For this review, take the finished solid that the model builds, in its own axes (mm). Face numbers are marked on the shaded views. A direction names the side the tool comes from. Give positions to 0.01 mm unless a question says otherwise; leave off trailing zeros. Write each loop counter-clockwise with the first axis right and the second up, starting at its lowest first coordinate (ties: lowest second). Pieces come first, ordered by that corner, then holes. Notation, with made-up numbers: (45, 36) -> (72, 36) arc R15 ccw to (72, 50) -> close; hole circle Ø6 at (-31, -4.75). An arc over 180 degrees is marked (long way). Return JSON: item names as keys, results as strings.
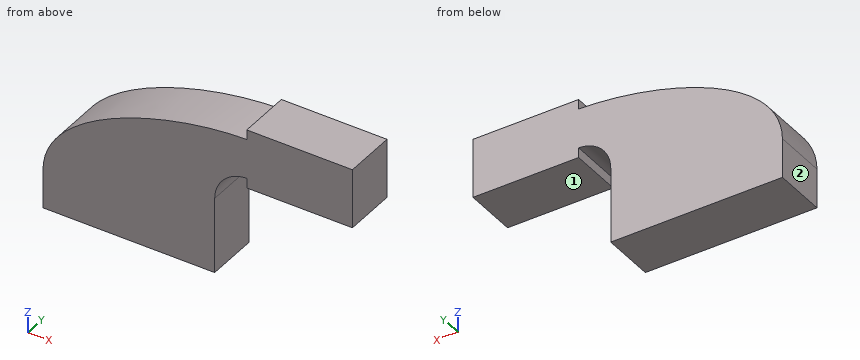
from build123d import *

# Parameters (mm, degrees)
F0_W     = 25.4
F0_H     = 28.575
F1_DEPTH = 25.4


with BuildPart() as f1:
    # F0 (on Front) → F1 (new body)
    with BuildSketch(Plane.XZ):
        Polygon((41.275, -9.525), (41.275, 9.525), (22.225, 9.525), (-41.275, 9.525), (-41.275, -9.525), align=None)
        with BuildLine():
            Line((22.225, 9.525), (41.275, 9.525))
            Line((41.275, 9.525), (41.275, 27.0002))
            ThreePointArc((41.275, 27.0002), (45.7700842218, 38.0687654844), (56.7097265362, 42.869093606))
            Line((56.7097265362, 42.869093606), (56.7097265362, 61.9219276004))
            add(Edge.make_bspline(
                [(56.5976430534, 61.9208318214), (56.6350247317, 61.9212149579), (56.6723859179, 61.921580219), (56.7097265362, 61.9219276004)],
                knots=[110.9664964384, 110.9664964384, 110.9664964384, 110.9664964384, 111.075437095, 111.075437095, 111.075437095, 111.075437095], degree=3))
            ThreePointArc((56.5976430534, 61.9208318214), (32.2597740934, 51.4998383508), (22.225, 27.0002))
            Line((22.225, 27.0002), (22.225, 9.525))
        make_face()
        with BuildLine():
            Line((-41.275, 9.525), (22.225, 9.525))
            Line((22.225, 9.525), (22.225, 27.0002))
            ThreePointArc((22.225, 27.0002), (32.2597740934, 51.4998383508), (56.5976430534, 61.9208318214))
            add(Edge.make_bspline(
                [(-41.275, 9.525), (-40.8172895576, 42.5938186475), (18.5208221845, 61.5305705249), (56.5976430534, 61.9208318214)],
                knots=[0, 0, 0, 0, 110.9664964384, 110.9664964384, 110.9664964384, 110.9664964384], degree=3))
        make_face()
        with BuildLine():
            Line((56.7097265362, 61.9219276004), (56.7097265362, 42.869093606))
            Line((56.7097265362, 42.869093606), (56.7097265362, 38.1))
            Line((56.7097265362, 38.1), (82.1097265362, 38.1))
            Line((82.1097265362, 38.1), (82.1097265362, 66.675))
            Line((82.1097265362, 66.675), (56.7097265362, 66.675))
            Line((56.7097265362, 66.675), (56.7097265362, 61.9224247899))
            ThreePointArc((56.7097265362, 61.9224247899), (56.9298588949, 61.9245061906), (57.15, 61.9252))
            add(Edge.make_bspline(
                [(56.7097265362, 61.9219276004), (56.856805001, 61.9232958778), (57.0035643669, 61.9243867627), (57.15, 61.9252)],
                knots=[111.075437095, 111.075437095, 111.075437095, 111.075437095, 111.5045361635, 111.5045361635, 111.5045361635, 111.5045361635], degree=3))
        make_face()
        with BuildLine():
            ThreePointArc((56.7097265362, 61.9224247899), (56.6536841557, 61.9216732734), (56.5976430534, 61.9208318214))
            add(Edge.make_bspline(
                [(56.5976430534, 61.9208318214), (56.6350247317, 61.9212149579), (56.6723859179, 61.921580219), (56.7097265362, 61.9219276004)],
                knots=[110.9664964384, 110.9664964384, 110.9664964384, 110.9664964384, 111.075437095, 111.075437095, 111.075437095, 111.075437095], degree=3))
            Line((56.7097265362, 61.9219276004), (56.7097265362, 61.9224247899))
        make_face()
        with BuildLine():
            Line((56.7097265362, 61.9224247899), (56.7097265362, 61.9219276004))
            add(Edge.make_bspline(
                [(56.7097265362, 61.9219276004), (56.856805001, 61.9232958778), (57.0035643669, 61.9243867627), (57.15, 61.9252)],
                knots=[111.075437095, 111.075437095, 111.075437095, 111.075437095, 111.5045361635, 111.5045361635, 111.5045361635, 111.5045361635], degree=3))
            ThreePointArc((57.15, 61.9252), (56.9298588949, 61.9245061906), (56.7097265362, 61.9224247899))
        make_face()
        with Locations((94.8097265362, 52.3875)):
            Rectangle(F0_W, F0_H)
    extrude(amount=F1_DEPTH)


solid = f1.part
1. For the marked faces 1 and 2, list the 3-axis set-ups (+Z, -Z, +X, -X, +Y, -Y) from which the entire face can be reached by the end or side of a thin tool; tool diameter is ignored.
Results found:
{"face 1": "-Z, +X, +Y, -Y", "face 2": "+Z, -Z, -X, +Y, -Y"}
2. To check wall thickness, follow probe 1 along Z at (x, y) = (93.5, -16) (3 decimals); probe 2 along X at (y, z) = (-6, 9.5) (3 decimals); probe 3 along X at (y, z) = (-9.5, 39). State the ranges of each line that lie inside material, in increasing order.
Results found:
{"probe 1": "z = 38.1 to 66.675", "probe 2": "x = -41.275 to 41.275", "probe 3": "x = -22.4 to 46.76, 56.71 to 107.51"}
3. Add section A-A, the plane z = 6. State the section outline as (x, y) points (3 decimals).
Results found:
{"outline": "(-41.275, -25.4) -> (41.275, -25.4) -> (41.275, 0) -> (-41.275, 0) -> close"}
4. Add section B-B, the plane x = 80. State the section outline as (y, z) points (3 decimals).
Results found:
{"outline": "(-25.4, 38.1) -> (0, 38.1) -> (0, 66.675) -> (-25.4, 66.675) -> close"}
5. For pin 1 (12 mm diameter, centred on x = 72, y = -16.5, fed in from -Z); pin 2 (4 mm diameter, centred on x = 47.5, y = -21.5, fed in from -Z); pin 3 (4 mm diameter, centred on y = -21.5, z = 11.5, fed in from +X) (3 decimals), all flat-tipped, find the tip position at first contact; note any pin that passes through.
Results found:
{"pin 1": "stops at z = 38.1", "pin 2": "stops at z = 37.78", "pin 3": "stops at x = 41.275"}
